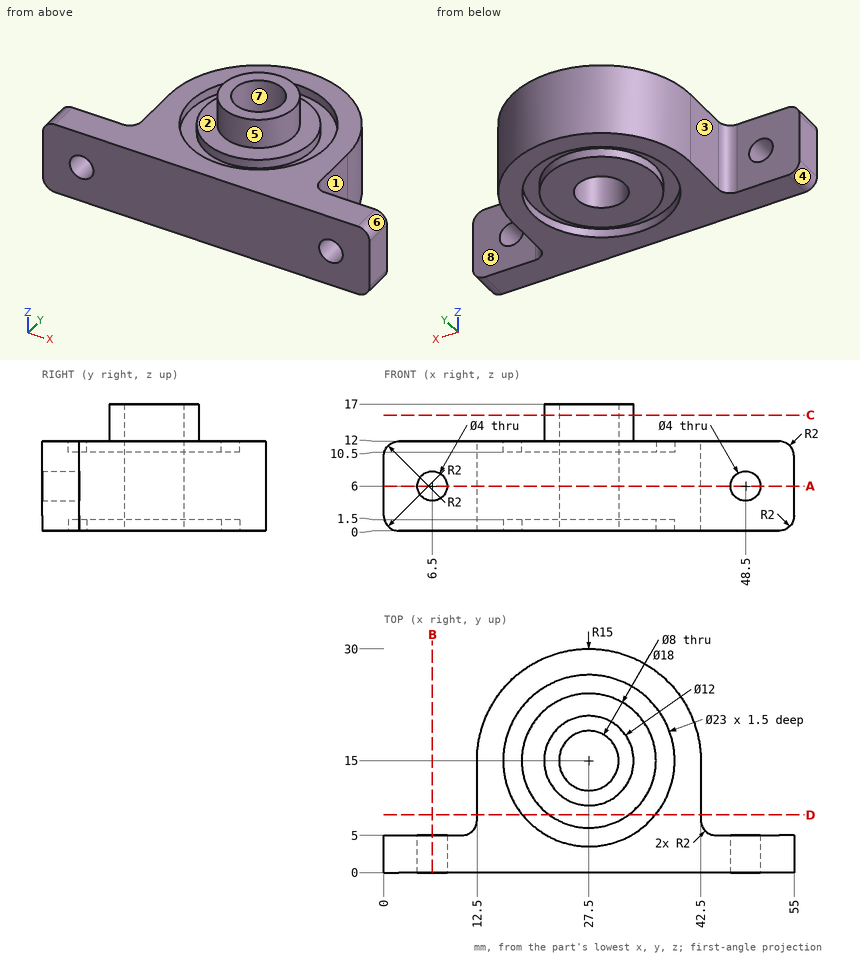
Check sheet for the drawn part. Datum: minimum x, y, z corner. Units: mm. A direction names the side the tool comes from. Round coordinates to 2 decimals unless told otherwise and drop trailing zeros. Loops run counter-clockwise (first coordinate to the right, second up) from the corner with the lowest first, then second, coordinate; pieces in that order, holes last. Notation, with made-up numbers: (48, 76) - (100, 76) arc R23 cw to (100, 105) - close; hole circle Ø8 at (78, 23). An arc over 180 degrees is marked (long way). Answer as a JSON object with one key per item and string values. Group by question number.
Q1. Sectioned sample at A-A, the plane z = 6. Enter the section's corners in (x, y), plus the area to 3 significant figures.
Q2. Gauge pin test, flat ends, axial feed: P1, Ø4.5, axis at x = 6.5, z = 6, coming from the +Y side; P2, Ø9, axis at x = 27.5, y = 15, coming from the +Z side; P3, Ø8, axis at y = 12.5, z = 6.5, coming from the +X side; P4, Ø3, axis at x = 32.5, z = 10.5, coming from the +Y side. Record the tip position at first contact, or that the pin passes through.
Q3. Set-up check for the marked faces 1, 2, 3 and 4: record each of +Z, -Z, +X, -X, +Y, -Y from which the full face is reachable in a straight line by a thin tool's end or side.
Q4. Sectioned sample at C-C, the plane z = 15.5. Enter the section's corners in (x, y).
Q5. Scan lines: line 1 along X through (y, z) = (2.4, 6); line 2 along Z through (x, y) = (6.5, 2.75); line 3 along Y through (x, z) = (27.5, 11). Record each from-to range of solid material in increasing order. Write a range as [from, to].
Q6. Mould release check, pull along Y, two halves, no side actions. Record for the marked faces 5, 6, 7 and 8: released by +Y, released by -Y, zero draft, split by the parting line, or undercut.
Q7. Sectioned sample at B-B, the plane x = 6.5. Enter the section's corners in (y, z), plus the area to 3 significant figures.
Q8. Sectioned sample at D-D, the plane y = 7.75. Enter the section's corners in (x, z), plus the area to 3 significant figures.
Solution:
{
 "1": {"outline": "(0, 0) - (4.5, 0) - (4.5, 5) - (0, 5) - close; (8.5, 0) - (46.5, 0) - (46.5, 5) - (44.5, 5) arc R2 cw to (42.5, 7) - (42.5, 15) arc R15 ccw to (12.5, 15) - (12.5, 7) arc R2 cw to (10.5, 5) - (8.5, 5) - close; (50.5, 0) - (55, 0) - (55, 5) - (50.5, 5) - close; hole circle Ø8 at (27.5, 15)", "area": "840 mm²"},
 "2": {"P1": "stops at y = 5", "P2": "stops at z = 17", "P3": "stops at x = 42.5", "P4": "stops at y = 29.59"},
 "3": {"face 1": "+Z, -Z, +X, +Y", "face 2": "+Z", "face 3": "+Z, -Z, -X, +Y", "face 4": "-Z, -X, +Y, -Y"},
 "4": {"outline": "circle Ø12 at (27.5, 15); hole circle Ø8 at (27.5, 15)"},
 "5": {"line 1": "x = [0, 4.5], [8.5, 46.5], [50.5, 55]", "line 2": "z = [0, 4], [8, 12]", "line 3": "y = [0, 3.5], [6, 11], [19, 24], [26.5, 30]"},
 "6": {"face 5": "split by the parting line", "face 6": "zero draft", "face 7": "undercut", "face 8": "released by +Y"},
 "7": {"outline": "(0, 0) - (5, 0) - (5, 4) - (0, 4) - close; (0, 8) - (5, 8) - (5, 12) - (0, 12) - close", "area": "40.0 mm²"},
 "8": {"outline": "(12.5, 0) - (18.57, 0) - (18.57, 1.5) - (22.17, 1.5) - (22.17, 0) - (32.83, 0) - (32.83, 1.5) - (36.43, 1.5) - (36.43, 0) - (42.5, 0) - (42.5, 12) - (36.43, 12) - (36.43, 10.5) - (32.83, 10.5) - (32.83, 12) - (22.17, 12) - (22.17, 10.5) - (18.57, 10.5) - (18.57, 12) - (12.5, 12) - close", "area": "338 mm²"}
}
